```python
from build123d import *

# Parameters (mm, degrees)
BOSS_EXTRUDE1_DEPTH      = 25
CUT_EXTRUDE2_DEPTH       = 194.321380264
SKETCH4_R                = 6.25
CUT_EXTRUDE5_DEPTH       = 3.5
SKETCH5_R                = 2.55
CUT_EXTRUDE6_DEPTH       = 194.321380264
SKETCH6_R                = 12.6
CUT_EXTRUDE7_DEPTH       = 194.321380264
SKETCH8_W                = 30
SKETCH8_H                = 12
BOSS_EXTRUDE2_DEPTH      = 25
FILLET1_R                = 15
FILLET2_R                = 2
CUT_EXTRUDE8_DEPTH       = 200.255045248
CUT_EXTRUDE8_DEPTH_BACK  = 200.255045248
SKETCH9_R                = 2.6
CUT_EXTRUDE9_START       = 2
SKETCH10_W               = 25
SKETCH10_H               = 16.5
CUT_EXTRUDE9_DEPTH       = 25
CUT_EXTRUDE10_START      = 28
SKETCH11_W               = 25
SKETCH11_H               = 16.5
CUT_EXTRUDE10_DEPTH      = 25
CUT_EXTRUDE11_DEPTH      = 200.255045248
CUT_EXTRUDE11_DEPTH_BACK = 200.255045248
SKETCH13_W               = 2.5
SKETCH13_H               = 16
FILLET6_R                = 7


with BuildPart() as part:
    # Sketch1 → Boss-Extrude1 (new body)
    with BuildSketch(Plane.XY):
        with BuildLine():
            Line((0, 0), (30, 0))
            Line((30, 0), (30, 150))
            ThreePointArc((30, 150), (15, 188.093476939), (0, 150))
            Line((0, 150), (0, 0))
        make_face()
    extrude(amount=BOSS_EXTRUDE1_DEPTH)

    # Sketch2 → Cut-Extrude2 (cut, through all)
    with BuildSketch(Plane(origin=(0, 0, 0), x_dir=(0, 0, -1), z_dir=(1, 0, 0))):
        Polygon((0, 0), (-25, 26), (-25, 0), align=None)
    extrude(amount=CUT_EXTRUDE2_DEPTH, mode=Mode.SUBTRACT)

    # Sketch4 → Cut-Extrude5 (cut)
    with BuildSketch(Plane.XY):
        with Locations((8, 13)):
            Circle(SKETCH4_R)
        with Locations((22, 13)):
            Circle(SKETCH4_R)
    extrude(amount=CUT_EXTRUDE5_DEPTH, mode=Mode.SUBTRACT)

    # Sketch5 → Cut-Extrude6 (cut, through all)
    with BuildSketch(Plane.XY):
        with Locations(Location((8, 13, 0), (0, 0, 270))):
            Circle(SKETCH5_R)
        with Locations(Location((22, 13, 0), (0, 0, 270))):
            Circle(SKETCH5_R)
    extrude(amount=CUT_EXTRUDE6_DEPTH, mode=Mode.SUBTRACT)

    # Sketch6 → Cut-Extrude7 (cut, through all)
    with BuildSketch(Plane.XY):
        with Locations((15, 166.093476939)):
            Circle(SKETCH6_R)
    extrude(amount=CUT_EXTRUDE7_DEPTH, mode=Mode.SUBTRACT)

    # Sketch8 → Boss-Extrude2 (add)
    with BuildSketch(Plane.XY):
        with Locations((15, 188.186953879)):
            Rectangle(SKETCH8_W, SKETCH8_H)
    extrude(amount=BOSS_EXTRUDE2_DEPTH)

    # Fillet1
    fillet1_edges = [part.edges().sort_by_distance(p)[0] for p in [
        (0, 182.186953879, 12.5),
        (30, 182.186953879, 12.5),
        (0, 150, 12.5),
        (30, 150, 12.5),
    ]]
    fillet(fillet1_edges, radius=FILLET1_R)

    # Fillet2
    fillet2_edges = [part.edges().sort_by_distance(p)[0] for p in [
        (0, 194.186953879, 12.5),
        (30, 194.186953879, 12.5),
    ]]
    fillet(fillet2_edges, radius=FILLET2_R)

    # Sketch9 → Cut-Extrude8 (cut, two sides: drawn at the far end of the back side and taken through both)
    with BuildSketch(Plane(origin=(0, 0, 0), x_dir=(0, 0, -1), z_dir=(1, 0, 0)).offset(-CUT_EXTRUDE8_DEPTH_BACK)):
        with Locations(Location((-6, 188.686953879, 0), (0, 0, 201.12545117))):
            Circle(SKETCH9_R)
        with Locations(Location((-19, 188.686953879, 0), (0, 0, 201.12545117))):
            Circle(SKETCH9_R)
    extrude(amount=CUT_EXTRUDE8_DEPTH + CUT_EXTRUDE8_DEPTH_BACK, mode=Mode.SUBTRACT)

    # Sketch10 → Cut-Extrude9 (cut)
    with BuildSketch(Plane(origin=(0, 0, 0), x_dir=(0, 0, -1), z_dir=(1, 0, 0)).offset(CUT_EXTRUDE9_START)):
        with Locations((-12.5, 190.936953879)):
            Rectangle(SKETCH10_W, SKETCH10_H)
    extrude(amount=-CUT_EXTRUDE9_DEPTH, mode=Mode.SUBTRACT)

    # Sketch11 → Cut-Extrude10 (cut)
    with BuildSketch(Plane(origin=(0, 0, 0), x_dir=(0, 0, -1), z_dir=(1, 0, 0)).offset(CUT_EXTRUDE10_START)):
        with Locations((-12.5, 190.936953879)):
            Rectangle(SKETCH11_W, SKETCH11_H)
    extrude(amount=CUT_EXTRUDE10_DEPTH, mode=Mode.SUBTRACT)

    # Sketch13 → Cut-Extrude11 (cut, two sides: drawn at the far end of the back side and taken through both)
    with BuildSketch(Plane.XY.offset(-CUT_EXTRUDE11_DEPTH_BACK)):
        with Locations((15, 186.186953879)):
            Rectangle(SKETCH13_W, SKETCH13_H)
    extrude(amount=CUT_EXTRUDE11_DEPTH + CUT_EXTRUDE11_DEPTH_BACK, mode=Mode.SUBTRACT)

    # Fillet6
    # the kernel refuses this fillet: 7 mm, written as the material it takes off along each edge
    with BuildSketch(Plane(origin=(30.880271574, 182.686953879, -8.501523298), x_dir=(-1, 0, 0), z_dir=(0, 0, 1))) as fillet6_piece_1:
        with BuildLine():
            CenterArc((4.384431788, 6.836483164), FILLET6_R, 212.743731737, 44.847779206)
            Line((-1.503255553, 3.050305966), (-1.6210093, 2.974582422))
            ThreePointArc((-1.6210093, 2.974582422), (-0.790485812, 1.506002918), (-0.131784132, -0.047254022))
            Line((-0.131784132, -0.047254022), (0, -0.14))
            ThreePointArc((0, -0.14), (1.440135787, -0.14), (2.85018837, -0.136729663))
            Line((2.85018837, -0.136729663), (2.880271574, 0))
        make_face()
    extrude(amount=42.003046595, mode=Mode.SUBTRACT)
    with BuildSketch(Plane(origin=(-0.880271574, 182.686953879, -8.501523298), x_dir=(-0.44205476486446993, -0.8969880628306143, 0), z_dir=(0, 0, 1))) as fillet6_piece_2:
        with BuildLine():
            CenterArc((4.194084827, 6.954882933), FILLET6_R, 218.64354594, 44.847779206)
            Line((-1.273237773, 2.58356922), (-1.382584225, 2.496142945))
            ThreePointArc((-1.382584225, 2.496142945), (-0.762197216, 1.229896943), (-0.125578329, -0.061887667))
            Line((-0.125578329, -0.061887667), (0.01586951, -0.139097659))
            ThreePointArc((0.01586951, -0.139097659), (1.70030466, -0.043320572), (3.384739809, -0.139097659))
            Line((3.384739809, -0.139097659), (3.400609319, 0))
        make_face()
    extrude(amount=42.003046595, mode=Mode.SUBTRACT)


solid = part.part
```
Geometry: final body of the model. Coordinates: model frame, mm. A direction names the side the tool comes from. Give positions to 0.01 mm unless a question says otherwise; leave off trailing zeros. Loops run counter-clockwise (first coordinate to the right, second up) from the corner with the lowest first, then second, coordinate; pieces in that order, holes last. Notation, with made-up numbers: (50.5, 16) - (77.5, 16) arc R22 ccw to (77.5, 50) - close; hole circle Ø9 at (63.5, 54). An arc over 180 degrees is marked (long way). Answer as CSV lines item,"result". Start each with the question number.
(1) Reachability of faces 4 (the face through (25, 13, 3.5)), 5 (the face through (37, 166, 12)), 6 (the face through (16.25, 186, 12)), 7 (the face through (30, 71, 12)), 8 (the face through (28, 189, 13)) from +Z, -Z, +X, -X, +Y, -Y: full face, straight path, thin tool, end or side. Return the list, or none.
(2) Section query D-D (y = 122.5). Output: boundary loops of the cut face in (x, z), and give its area (3 significant figures).
(3) Section query B-B (x = 8). Output: boundary loops of the cut face in (y, z).
(4) Pin query (flat end, axial travel): P1, Ø9, axis at y = 191, z = 12, coming from the -X side; P2, Ø8, axis at x = 6.5, z = 9.5, coming from the -Y side; P3, Ø7.5, axis at y = 95, z = 11, coming from the +X side. Return the tip coordinate at first contact, or that it passes through.
(5) Section query C-C (z = 19). Output: boundary loops of the cut face in (x, y), and give its area (3 significant figures).
(6) Ray query, line 1 along X through (y, z) = (13, 11.5); line 2 along Y through (x, z) = (12.5, 5.5); line 3 along Y through (x, z) = (8, 2.55). Return the intervals inside material, ascending. Write a range as [from, to].
(7) Mould query, pull axis X, two halves, no side actions, for faces 1 (the face through (13.75, 186, 12)), 2 (the face through (-7, 166, 12)), 3 (the face through (15, 111, 25)). Classes: +X half, -X half, draft (parallel to the pull), parting line (faces both ways), or undercut.
(8) Section query A-A (z = 6). Output: boundary loops of the cut face in (x, y), and give its area (3 significant figures).
Worked answers:
1,face 4,"-Z"
1,face 5,"+Z, -Z, +X"
1,face 6,"+Z, -Z, +Y"
1,face 7,"+Z, -Z, +X, -Y"
1,face 8,"+Z, -Z, +X, +Y"
2,outline,"(0, 0) - (30, 0) - (30, 25) - (0, 25) - close"
2,area,"750 mm^2"
3,outline,"(0, 0) - (6.75, 0) - (6.75, 3.5) - (10.45, 3.5) - (10.45, 10.05) - close; (15.55, 3.5) - (19.25, 3.5) - (19.25, 0) - (155.62, 0) - (155.62, 25) - (26, 25) - (15.55, 14.95) - close; (176.57, 0) - (194.19, 0) - (194.19, 25) - (176.57, 25) - close; hole circle Ø5.2 at (188.69, 6); hole circle Ø5.2 at (188.69, 19)"
4,P1,"stops at x = 2"
4,P2,"stops at y = 5.72"
4,P3,"stops at x = 30"
5,outline,"(-2.84, 153.22) arc R15 cw to (0, 144.44) - (0, 19.76) - (30, 19.76) - (30, 144.44) arc R15 cw to (32.84, 153.22) arc R22 ccw to (32.84, 178.97) arc R15 cw to (32.38, 179.64) arc R7 ccw to (28, 182.69) - (28, 186.09) - (16.25, 186.09) - (16.25, 178.63) arc R12.6 cw (long way) to (13.75, 178.63) - (13.75, 186.09) - (2, 186.09) - (2, 182.69) arc R7 ccw to (-2.38, 179.64) arc R15 cw to (-2.84, 178.97) arc R22 ccw to start; (2, 191.29) - (13.75, 191.29) - (13.75, 194.19) - (2, 194.19) - close; (16.25, 191.29) - (28, 191.29) - (28, 194.19) - (16.25, 194.19) - close"
5,area,"4,840 mm^2"
6,line 1,"x = [0, 5.45], [10.55, 19.45], [24.55, 30]"
6,line 2,"y = [5.72, 153.74], [178.44, 186.14], [191.24, 194.19]"
6,line 3,"y = [2.65, 6.75], [19.25, 155.62], [176.57, 194.19]"
7,face 1,"undercut"
7,face 2,"-X half"
7,face 3,"draft"
8,outline,"(-2.84, 153.22) arc R15 cw to (0, 144.44) - (0, 6.24) - (30, 6.24) - (30, 144.44) arc R15 cw to (32.84, 153.22) arc R22 ccw to (32.84, 178.97) arc R15 cw to (32.38, 179.64) arc R7 ccw to (28, 182.69) - (28, 186.09) - (16.25, 186.09) - (16.25, 178.63) arc R12.6 cw (long way) to (13.75, 178.63) - (13.75, 186.09) - (2, 186.09) - (2, 182.69) arc R7 ccw to (-2.38, 179.64) arc R15 cw to (-2.84, 178.97) arc R22 ccw to start; (2, 191.29) - (13.75, 191.29) - (13.75, 194.19) - (2, 194.19) - close; (16.25, 191.29) - (28, 191.29) - (28, 194.19) - (16.25, 194.19) - close; hole circle Ø5.1 at (8, 13); hole circle Ø5.1 at (22, 13)"
8,area,"5,210 mm^2"
